For this review, take the finished solid that the model builds, in its own axes (mm). A direction names the side the tool comes from. Round coordinates to 2 decimals unless told otherwise and drop trailing zeros. Write each loop counter-clockwise with the first axis right and the second up, starting at its lowest first coordinate (ties: lowest second). Pieces come first, ordered by that corner, then holes. Notation, with made-up numbers: (63, 64) - (99, 64) arc R7 cw to (99, 69) - close; hole circle Ø10 at (68.25, -34.75). An arc over 180 degrees is marked (long way). Answer in a Markdown table with one row per item. Add a question column.
from build123d import *

# Parameters (mm, degrees)
F1_DEPTH      = 47.752
F2_W          = 39.37
F2_H          = 39.37
F3_DEPTH      = 8.382
F4_R          = 88.9
F4_R_2        = 6.35
F5_DEPTH      = 12.7
F7_DEPTH      = 50.8
F8_R          = 5.334
F9_DEPTH      = 88.901
F9_DEPTH_BACK = 127
F10_W         = 36.83
F10_H         = 36.83
F11_DEPTH     = 50.8
F13_DEPTH     = 34.925
F14_W         = 139.7
F14_H         = 44.45
F15_DEPTH     = 252.932645439
F17_DEPTH     = 22.225
F18_R         = 5.08
F19_R         = 6.35
F20_DEPTH     = 123.826


with BuildPart() as f1:
    # F0 (on Top) → F1 (new body)
    with BuildSketch(Plane.XY):
        with BuildLine():
            Line((-4.7625, 15.4178), (-4.7625, 18.1826348407))
            ThreePointArc((-4.7625, 18.1826348407), (0, -18.796), (4.7625, 18.1826348407))
            Line((4.7625, 18.1826348407), (4.7625, 15.4178))
            Line((4.7625, 15.4178), (-4.7625, 15.4178))
        make_face()
    extrude(amount=F1_DEPTH)

    # F2 (on face) → F3 (join)
    with BuildSketch(Plane.XY.offset(47.752)):
        Rectangle(F2_W, F2_H)
    extrude(amount=F3_DEPTH)

    # F4 (on face) → F5 (join)
    with BuildSketch(Plane.XY.offset(56.134)):
        Circle(F4_R)
        with Locations((-54.9926131403, -31.75)):
            Circle(F4_R_2, mode=Mode.SUBTRACT)
        with Locations((0, -63.5)):
            Circle(F4_R_2, mode=Mode.SUBTRACT)
        with Locations((54.9926131403, -31.75)):
            Circle(F4_R_2, mode=Mode.SUBTRACT)
        with Locations((-54.9926131403, 31.75)):
            Circle(F4_R_2, mode=Mode.SUBTRACT)
        with Locations((54.9926131403, 31.75)):
            Circle(F4_R_2, mode=Mode.SUBTRACT)
        with Locations((0, 63.5)):
            Circle(F4_R_2, mode=Mode.SUBTRACT)
    extrude(amount=F5_DEPTH)

    # F6 (on face) → F7 (join)
    with BuildSketch(Plane.XY.offset(68.834)):
        with BuildLine():
            Line((27.305, 31.115), (-27.305, 31.115))
            ThreePointArc((-27.305, 31.115), (-29.9990768363, 29.9990768363), (-31.115, 27.305))
            Line((-31.115, 27.305), (-31.115, -27.305))
            ThreePointArc((-31.115, -27.305), (-29.9990768363, -29.9990768363), (-27.305, -31.115))
            Line((-27.305, -31.115), (27.305, -31.115))
            ThreePointArc((27.305, -31.115), (29.9990768363, -29.9990768363), (31.115, -27.305))
            Line((31.115, -27.305), (31.115, 27.305))
            ThreePointArc((31.115, 27.305), (29.9990768363, 29.9990768363), (27.305, 31.115))
        make_face()
    extrude(amount=F7_DEPTH)

    # F8 (on Right) → F9 (cut, two sides)
    with BuildSketch(Plane.YZ) as f9_sk:
        with Locations((0, 31.75)):
            Circle(F8_R)
    extrude(amount=F9_DEPTH, mode=Mode.SUBTRACT)
    extrude(f9_sk.sketch, amount=-F9_DEPTH_BACK, mode=Mode.SUBTRACT)

    # F10 (on face) → F11 (cut, through all)
    with BuildSketch(Plane.XY.offset(119.634)):
        Rectangle(F10_W, F10_H)
    extrude(amount=-F11_DEPTH, mode=Mode.SUBTRACT)

    # F12 (on Front) → F13 (join, symmetric)
    with BuildSketch(Plane.XZ):
        Polygon((0, 119.634), (31.115, 119.634), (82.55, 184.201354561), (82.55, 437.134), (38.354, 437.134), (38.354, 373.634), (0, 373.634), (-38.354, 373.634), (-38.354, 437.134), (-82.55, 437.134), (-82.55, 184.201354561), (-31.115, 119.634), align=None)
    extrude(amount=F13_DEPTH, both=True)

    # F14 (on face) → F15 (cut, through all)
    with BuildSketch(Plane.XY.offset(437.134)):
        Rectangle(F14_W, F14_H)
    extrude(amount=-F15_DEPTH, mode=Mode.SUBTRACT)

    # F16 (on Front) → F17 (cut, symmetric)
    with BuildSketch(Plane.XZ):
        Polygon((31.115, 140.0167160494), (66.3129246679, 184.201354561), (-66.3129246679, 184.201354561), (-31.115, 140.0167160494), (-18.415, 140.0167160494), (-18.415, 68.834), (18.415, 68.834), (18.415, 140.0167160494), align=None)
    extrude(amount=F17_DEPTH, both=True, mode=Mode.SUBTRACT)

    # F18
    f18_edges = [f1.edges().sort_by_distance(p)[0] for p in [
        (82.55, 0, 184.201355),
        (-82.55, 0, 184.201355),
    ]]
    fillet(f18_edges, radius=F18_R)

    # F19 (on face) → F20 (cut, through all)
    with BuildSketch(Plane.XZ.offset(34.925)):
        with Locations((0, 189.484)):
            Circle(F19_R)
        with Locations((0, 268.859)):
            Circle(F19_R)
    extrude(amount=-F20_DEPTH, mode=Mode.SUBTRACT)


solid = f1.part
Q1. Add section D-D on y = 63.5. State the section outline as (x, z) points, then the cut area to 3 significant figures.
Q2. Add section B-B on z = 409.5. State the section outline as (x, y) points (3 decimals), then the cut area to 3 significant figures.
Q3. To check wall thickness, follow probe 1 along Y at (x, z) = (19.5, 253.5) (3 decimals); probe 2 along X at (y, z) = (-18.5, 390); probe 3 along Y at (x, z) = (10, 109) (3 decimals). State the ranges of each line that lie inside material, in increasing order.
Q4. Add section A-A on z = 299. State the section outline as (x, y) points (3 decimals).
Q5. Insertion check: pin 1 Ø10 at (x, y) = (2, 30.5) entering from +Z; pin 2 Ø10 at (x, z) = (68.5, 258) entering from +Y (3 decimals); pin 3 Ø9 at (y, z) = (7, 54) entering from +X. Each pin has a flat end and moves straight along its axis. Give the tip position at first contact, or say it passes through.
Q6. Tool access review of faces 5 (the face through (-1, -34.925, 281)), 6 (the face through (-19.685, 0, 52)), 7 (the face through (0, -19.685, 52)): name each direction out of +Z, -Z, +X, -X, +Y, -Y from which nothing blocks a thin tool from reaching the whole face with its end or side.
Q7. Draft analysis for pull direction X (two halves, no side actions). For faces 1 (the face through (-1.377, -28.664, 183.285)), 2 (the face through (-82.55, 0, 313)), 3 (the face through (-1, -38, 68.834)), 4 (the face through (18.415, 0, 104)), state which applies: released by +X, released by -X, zero draft, split by the parting line, or undercut.
Q8. Add section C-C on x = 0. Count the separate pieces of the cut face and the enclosed holes in it, then the cut area to 3 significant figures.
Answer sheet:
| question | item | result |
|---|---|---|
| 1 | outline | (-62.22, 56.13) - (-6.35, 56.13) - (-6.35, 68.83) - (-62.22, 68.83) - close; (6.35, 56.13) - (62.22, 56.13) - (62.22, 68.83) - (6.35, 68.83) - close |
| 1 | area | 1,420 mm² |
| 2 | outline | (-82.55, -34.925) - (-38.354, -34.925) - (-38.354, -22.225) - (-69.85, -22.225) - (-69.85, 22.225) - (-38.354, 22.225) - (-38.354, 34.925) - (-82.55, 34.925) - close; (38.354, -34.925) - (82.55, -34.925) - (82.55, 34.925) - (38.354, 34.925) - (38.354, 22.225) - (69.85, 22.225) - (69.85, -22.225) - (38.354, -22.225) - close |
| 2 | area | 3,370 mm² |
| 3 | probe 1 | y = -34.925 to -22.225, 22.225 to 34.925 |
| 3 | probe 2 | x = -82.55 to -69.85, 69.85 to 82.55 |
| 3 | probe 3 | y = -31.115 to -22.225, 22.225 to 31.115 |
| 4 | outline | (-82.55, -34.925) - (82.55, -34.925) - (82.55, 34.925) - (-82.55, 34.925) - close; hole (-69.85, -22.225) - (69.85, -22.225) - (69.85, 22.225) - (-69.85, 22.225) - close |
| 5 | pin 1 | stops at z = 373.63 |
| 5 | pin 2 | stops at y = 34.925 |
| 5 | pin 3 | stops at x = 88.85 |
| 6 | face 5 | +Z, +X, -X, -Y |
| 6 | face 6 | -Z, -X, +Y, -Y |
| 6 | face 7 | -Z, +X, -X, -Y |
| 7 | face 1 | undercut |
| 7 | face 2 | released by -X |
| 7 | face 3 | zero draft |
| 7 | face 4 | undercut |
| 8 | separate pieces | 7 |
| 8 | enclosed holes | 1 |
| 8 | area | 10,500 mm² |
